Geometry: see drawing. Coordinates: mm, zero at the bounding-box minimum. Coordinates: 2 decimals unless noted, no trailing zeros. Write each loop counter-clockwise with the first axis right and the second up, starting at its lowest first coordinate (ties: lowest second). Pieces come first, ordered by that corner, then holes. Notation, with made-up numbers: (-38.75, 43) - (-24.75, 43) arc R18 cw to (-24.75, 67) - close; hole circle Ø8 at (24.5, 68.25). An arc over 180 degrees is marked (long way). One line per question, with ' | ' between items. Start each with the question number.
1) Draft query along X for the marked faces 1, 2, 3 and 4. Return one class per face: released by +X, released by -X, zero draft, split by the parting line, or undercut.
2) Section query C-C on y = 1.75. Return loops of the section in (x, z), and give its area (3 significant figures).
3) Section query A-A on x = 4. Return loops of the section in (y, z).
4) Section query B-B on z = 3.75. Return loops of the section in (x, y).
5) Line query: line 1 (X direction, y = 0.9, z = 3.75); line 2 (Z direction, x = 17, y = 1.35); line 3 (X direction, y = 1.55, z = 4.5). Output: solid intervals per line, ascending.
6) Section query D-D on x = 17.25. Return loops of the section in (y, z), and give its area (3 significant figures).
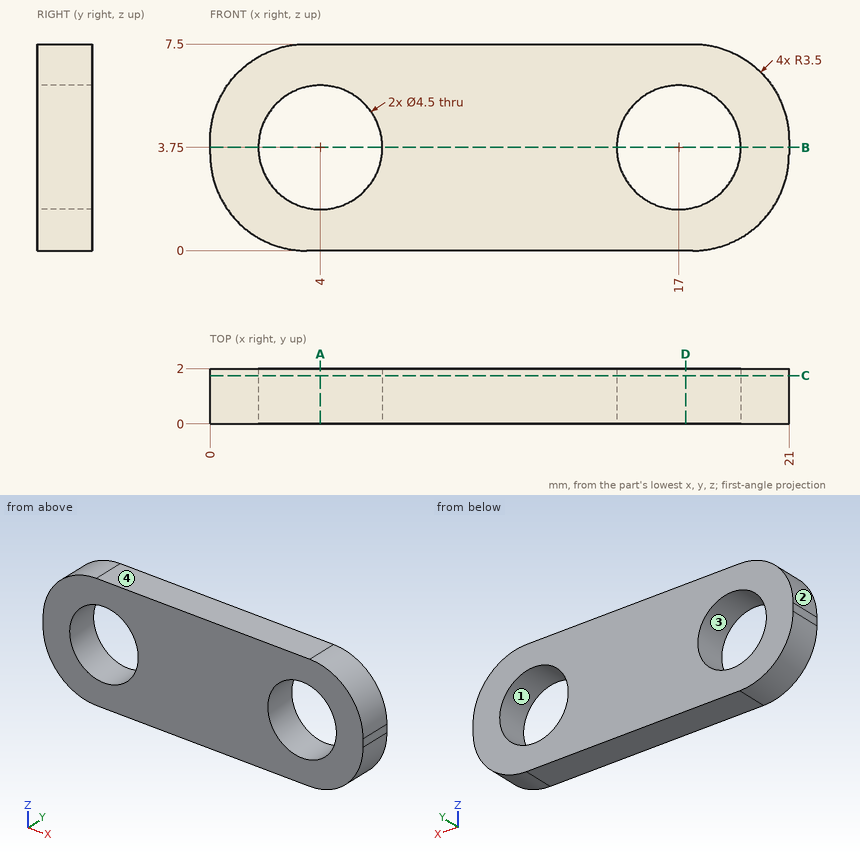
Answer key:
1) face 1: undercut | face 2: released by -X | face 3: undercut | face 4: zero draft
2) outline: (0, 3.5) arc R3.5 ccw to (3.5, 0) - (17.5, 0) arc R3.5 ccw to (21, 3.5) - (21, 4) arc R3.5 ccw to (17.5, 7.5) - (3.5, 7.5) arc R3.5 ccw to (0, 4) - close; hole circle Ø4.5 at (4, 3.75); hole circle Ø4.5 at (17, 3.75) | area: 115 mm²
3) outline: (0, 0) - (2, 0) - (2, 1.5) - (0, 1.5) - close; (0, 6) - (2, 6) - (2, 7.5) - (0, 7.5) - close
4) outline: (0, 0) - (1.75, 0) - (1.75, 2) - (0, 2) - close; (6.25, 0) - (14.75, 0) - (14.75, 2) - (6.25, 2) - close; (19.25, 0) - (21, 0) - (21, 2) - (19.25, 2) - close
5) line 1: 0 to 1.75, 6.25 to 14.75, 19.25 to 21 | line 2: 0 to 1.5, 6 to 7.5 | line 3: 0.04 to 1.88, 6.12 to 14.88, 19.12 to 20.96
6) outline: (0, 0) - (2, 0) - (2, 1.51) - (0, 1.51) - close; (0, 5.99) - (2, 5.99) - (2, 7.5) - (0, 7.5) - close | area: 6.06 mm²
